Build history of the part. All positions in model axes, mm. Round coordinates to 2 decimals unless told otherwise and drop trailing zeros. Write each loop counter-clockwise with the first axis right and the second up, starting at its lowest first coordinate (ties: lowest second). Pieces come first, ordered by that corner, then holes.
Item 1: Mould opens along Y. For faces 1 (the cylindrical face through (60.63, -59.49, 92.15)), 2 (the flat face through (48, -1, 95)), 3 (the cylindrical face through (65, 0, -1)) say: +Y half, -Y half, draft (parallel to the pull), parting line (faces both ways), or undercut.
Item 2: Band-saw the part on C-C, the plane z = 61. Write the cut outline in (x, y).
Item 3: Band-saw the part on B-B, the plane x = 60. Write the cut outline in (y, z).
Item 4: Drop a flat-ended pin along its axis: pin 1 Ø6 at (x, y) = (60, 0) entering from +Z. Give the stop position or say it passes through.
Item 5: Band-saw the part on A-A, the plane y = 0. Write the cut outline in (x, z), then the cut area to 3 significant figures.
Item 6: Wall check: probe 1 along Y at (x, z) = (60, 48); probe 2 along X at (y, z) = (-36, 87.5); probe 3 along Y at (x, z) = (114, 42.5). Give the ranges that are in metal, low to high.
```python
from build123d import *

# Parameters (mm, degrees)
SCHIZZO2_W                   = 190
SCHIZZO2_H                   = 125
ESTRUSIONE_ESTRUSIONE1_DEPTH = 120
RACCORDO1_R                  = 15
RACCORDO2_R                  = 10
SCHIZZO3_R                   = 5
TAGLIO_ESTRUSIONE1_DEPTH     = 191


with BuildPart() as part:
    # Schizzo2 → Estrusione-Estrusione1 (new body)
    with BuildSketch(Plane(origin=(0, 0, 0), x_dir=(0, 0, -1), z_dir=(1, 0, 0))):
        Rectangle(SCHIZZO2_W, SCHIZZO2_H)
    extrude(amount=ESTRUSIONE_ESTRUSIONE1_DEPTH)

    # Raccordo1
    raccordo1_edges = [part.edges().sort_by_distance(p)[0] for p in [
        (120, -62.5, 0),
        (0, -62.5, 0),
        (0, 62.5, 0),
        (120, 62.5, 0),
    ]]
    fillet(raccordo1_edges, radius=RACCORDO1_R)

    # Raccordo2
    raccordo2_edges = [part.edges().sort_by_distance(p)[0] for p in [
        (120, 0, 95),
        (0, 0, 95),
        (60, -62.5, 95),
        (60, 62.5, 95),
        (4.393398282, -58.106601718, 95),
        (4.393398282, 58.106601718, 95),
        (115.606601718, -58.106601718, 95),
        (115.606601718, 58.106601718, 95),
    ]]
    fillet(raccordo2_edges, radius=RACCORDO2_R)

    # Schizzo3 → Taglio-Estrusione1 (cut, through all)
    with BuildSketch(Plane(origin=(0, 0, -95), x_dir=(-1, 0, 0), z_dir=(0, 0, -1))):
        with Locations((-60, 0)):
            Circle(SCHIZZO3_R)
    extrude(amount=-TAGLIO_ESTRUSIONE1_DEPTH, mode=Mode.SUBTRACT)


solid = part.part
```
Results:
1. face 1: -Y half
1. face 2: draft
1. face 3: undercut
2. outline: (0, -47.5) arc R15 ccw to (15, -62.5) - (105, -62.5) arc R15 ccw to (120, -47.5) - (120, 47.5) arc R15 ccw to (105, 62.5) - (15, 62.5) arc R15 ccw to (0, 47.5) - close; hole circle Ø10 at (60, 0)
3. outline: (-62.5, -95) - (-5, -95) - (-5, 95) - (-52.5, 95) arc R10 ccw to (-62.5, 85) - close; (5, -95) - (62.5, -95) - (62.5, 85) arc R10 ccw to (52.5, 95) - (5, 95) - close
4. pin 1: passes through
5. outline: (0, -95) - (55, -95) - (55, 95) - (10, 95) arc R10 ccw to (0, 85) - close; (65, -95) - (120, -95) - (120, 85) arc R10 ccw to (110, 95) - (65, 95) - close
5. area: 20,900 mm2
6. probe 1: y = -62.5 to -5, 5 to 62.5
6. probe 2: x = 0.32 to 119.68
6. probe 3: y = -59.5 to 59.5
